```python
from build123d import *

# Parameters (mm, degrees)
SKETCH1_W           = 14
SKETCH1_H           = 14
BOSS_EXTRUDE1_DEPTH = 23.4
SKETCH2_W           = 14
SKETCH2_H           = 14
SKETCH2_W_2         = 8.8
SKETCH2_H_2         = 8.8
CUT_EXTRUDE1_DEPTH  = 3.4
SKETCH3_W           = 14
SKETCH3_H           = 14
SKETCH3_W_2         = 12
SKETCH3_H_2         = 10.9
CUT_EXTRUDE2_DEPTH  = 17.5
SKETCH4_W           = 12
SKETCH4_H           = 10.9
SKETCH4_W_2         = 0.5
SKETCH4_H_2         = 3.2
CUT_EXTRUDE3_DEPTH  = 5.5
CHAMFER1_SIZE       = 1.25


with BuildPart() as part:
    # Sketch1 → Boss-Extrude1 (new body)
    with BuildSketch(Plane.XY):
        Rectangle(SKETCH1_W, SKETCH1_H)
    extrude(amount=BOSS_EXTRUDE1_DEPTH)

    # Sketch2 → Cut-Extrude1 (cut)
    with BuildSketch(Plane.XY.offset(23.4)):
        Rectangle(SKETCH2_W, SKETCH2_H)
        Rectangle(SKETCH2_W_2, SKETCH2_H_2, mode=Mode.SUBTRACT)
    extrude(amount=-CUT_EXTRUDE1_DEPTH, mode=Mode.SUBTRACT)

    # Sketch3 → Cut-Extrude2 (cut)
    with BuildSketch(Plane(origin=(0, 0, 0), x_dir=(-1, 0, 0), z_dir=(0, 0, -1))):
        Rectangle(SKETCH3_W, SKETCH3_H)
        Rectangle(SKETCH3_W_2, SKETCH3_H_2, mode=Mode.SUBTRACT)
    extrude(amount=-CUT_EXTRUDE2_DEPTH, mode=Mode.SUBTRACT)

    # Sketch4 → Cut-Extrude3 (cut)
    with BuildSketch(Plane(origin=(0, 0, 0), x_dir=(-1, 0, 0), z_dir=(0, 0, -1))):
        Rectangle(SKETCH4_W, SKETCH4_H)
        with Locations((-3.25, 0)):
            Rectangle(SKETCH4_W_2, SKETCH4_H_2, mode=Mode.SUBTRACT)
        with Locations((3.25, 0)):
            Rectangle(SKETCH4_W_2, SKETCH4_H_2, mode=Mode.SUBTRACT)
    extrude(amount=-CUT_EXTRUDE3_DEPTH, mode=Mode.SUBTRACT)

    # Chamfer1
    chamfer1_edges = [part.edges().sort_by_distance(p)[0] for p in [
        (-7, 0, 20),
        (0, 7, 20),
        (7, 0, 20),
        (0, -7, 20),
    ]]
    chamfer(chamfer1_edges, length=CHAMFER1_SIZE)


solid = part.part
```
Source: CAD feature listing. Evaluate the final solid. Frame: model axes, mm. A direction names the side the tool comes from. Give positions to 0.01 mm unless a question says otherwise; leave off trailing zeros. Order: outer loops, then holes, each group sorted by start corner. A loop starts at its lowest first (then second) coordinate and runs counter-clockwise, first axis right, second up.
(1) Section query D-D (y = -4). Return the cut outline in (x, z), plus the area to 3 significant figures.
(2) Material intervals for line 1 along X through (y, z) = (4.25, 6); line 2 along Z through (x, y) = (2.25, 4.5); line 3 along Z through (x, y) = (3, 2.25), sorted ascending.
(3) Section query B-B (y = 1). Return the cut outline in (x, z).
(4) Section query C-C (x = 5.5). Return the cut outline in (y, z).
(5) Access query for faces 1 (the face through (4.4, 0, 22)), 2 (the face through (3, 0, 3)), 3 (the face through (3.5, 0, 3)). Directions: +Z, -Z, +X, -X, +Y, -Y. A direction counts if a zero-diameter tool reaches every point of the face in a straight line with its end or side. Return the directions, or none.
(6) Contact query for flat-ended pins moving along their axis: P1, Ø2, axis at x = 4, z = 13.5, coming from the +Y side; P2, Ø3.5, axis at x = 1, z = 11.5, coming from the -Y side; P3, Ø1, axis at x = 4, y = -4, coming from the -Z side. Output: stop coordinate, or through.
(7) Section query A-A (z = 1.5). Return the cut outline in (x, y).
Outcome:
1. outline: (-7, 17.5) - (-6, 17.5) - (-6, 5.5) - (6, 5.5) - (6, 17.5) - (7, 17.5) - (7, 18.75) - (5.75, 20) - (4.4, 20) - (4.4, 23.4) - (-4.4, 23.4) - (-4.4, 20) - (-5.75, 20) - (-7, 18.75) - close
1. area: 207 mm2
2. line 1: x = -6 to 6
2. line 2: z = 5.5 to 20
2. line 3: z = 5.5 to 23.4
3. outline: (-7, 17.5) - (-6, 17.5) - (-6, 5.5) - (-3.5, 5.5) - (-3.5, 0) - (-3, 0) - (-3, 5.5) - (3, 5.5) - (3, 0) - (3.5, 0) - (3.5, 5.5) - (6, 5.5) - (6, 17.5) - (7, 17.5) - (7, 18.75) - (5.75, 20) - (4.4, 20) - (4.4, 23.4) - (-4.4, 23.4) - (-4.4, 20) - (-5.75, 20) - (-7, 18.75) - close
4. outline: (-7, 17.5) - (-5.45, 17.5) - (-5.45, 5.5) - (5.45, 5.5) - (5.45, 17.5) - (7, 17.5) - (7, 18.75) - (5.75, 20) - (-5.75, 20) - (-7, 18.75) - close
5. face 1: +Z, +X, +Y, -Y
5. face 2: -Z, +Y, -Y
5. face 3: -Z, +X, +Y, -Y
6. P1: stops at y = 5.45
6. P2: stops at y = -5.45
6. P3: stops at z = 5.5
7. outline: (-3.5, -1.6) - (-3, -1.6) - (-3, 1.6) - (-3.5, 1.6) - close; (3, -1.6) - (3.5, -1.6) - (3.5, 1.6) - (3, 1.6) - close
